For this review, take the finished solid that the model builds, in its own axes (mm). Round coordinates to 2 decimals unless told otherwise and drop trailing zeros. Write each loop counter-clockwise with the first axis right and the second up, starting at its lowest first coordinate (ties: lowest second). Pieces come first, ordered by that corner, then holes. Notation, with made-up numbers: M 11.25,60 L 56.25,60 A13 ccw 56.25,74 Z; hole C 84,32 d11. An arc over 180 degrees is marked long. Use one line per item in the form item = value. Start each with the question number.
Item 1: For line 1 (Y direction, x = -55, z = -0.85); line 2 (X direction, y = -1, z = -4.5); line 3 (Y direction, x = -48, z = -6.5), list the stretches that pass through material, from the lowest coordinate up. Write a range as [from, to].
Item 2: Add section C-C (z = -7.5). State the section outline as (x, y) points, and give its area (3 significant figures).
Item 3: Add section B-B (x = -19.5). State the section outline as (y, z) points, and give its area (3 significant figures).
Item 4: For P1, Ø5, axis at y = 2, z = -7.5, coming from the -X side; P2, Ø6, axis at x = -37.5, y = -3.5, coming from the +Z side; P3, Ø0.8, axis at x = 28.5, z = 0.5, coming from the -Y side, all flat-tipped, find the tip position at first contact; note any pin that passes through.
Item 5: Add section A-A (y = -1). State the section outline as (x, z) points.
Item 6: Add section D-D (y = 3.25). State the section outline as (x, z) points, and give its area (3 significant figures).
from build123d import *

# Parameters (mm, degrees)
F0_R     = 2.25
F0_W     = 15
F0_H     = 4.4
F1_DEPTH = 3
F2_DEPTH = 1.5
F4_DEPTH = 50


with BuildPart() as f1:
    # F0 (on Top) → F1 (new body)
    with BuildSketch(Plane.XY):
        with BuildLine():
            ThreePointArc((-50, 0), (-51.464466, 3.535534), (-55, 5))
            ThreePointArc((-55, 5), (-60, 0), (-55, -5))
            ThreePointArc((-55, -5), (-51.464466, -3.535534), (-50, 0))
        make_face()
        with Locations((-55, 0)):
            Circle(F0_R, mode=Mode.SUBTRACT)
        with BuildLine():
            ThreePointArc((55, -5), (50, 0), (55, 5))
            Line((55, 5), (-55, 5))
            ThreePointArc((-55, 5), (-51.464466, 3.535534), (-50, 0))
            ThreePointArc((-50, 0), (-51.464466, -3.535534), (-55, -5))
            Line((-55, -5), (55, -5))
        make_face()
        with Locations((-25, 0)):
            Rectangle(F0_W, F0_H, mode=Mode.SUBTRACT)
        with Locations((25, 0)):
            Rectangle(F0_W, F0_H, mode=Mode.SUBTRACT)
        with Locations((-25, 0)):
            Rectangle(F0_W, F0_H)
        with Locations((25, 0)):
            Rectangle(F0_W, F0_H)
        with BuildLine():
            ThreePointArc((55, -5), (58.535534, -3.535534), (60, 0))
            ThreePointArc((60, 0), (58.535534, 3.535534), (55, 5))
            ThreePointArc((55, 5), (50, 0), (55, -5))
        make_face()
        with Locations((55, 0)):
            Circle(F0_R, mode=Mode.SUBTRACT)
    extrude(amount=-F1_DEPTH)

    # F0 (on Top) → F2 (join)
    with BuildSketch(Plane.XY):
        with Locations((-25, 0)):
            Rectangle(F0_W, F0_H)
        with Locations((25, 0)):
            Rectangle(F0_W, F0_H)
    extrude(amount=F2_DEPTH)

    # F3 (on Right) → F4 (join, symmetric)
    with BuildSketch(Plane.YZ):
        Polygon((5, -3), (-5, -3), (-5, -13), align=None)
    extrude(amount=F4_DEPTH, both=True)


solid = f1.part
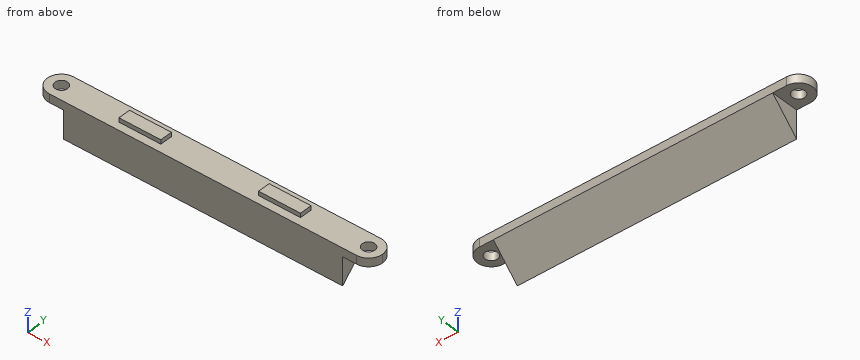
Calculated:
q1.line_1 = [-5, -2.25], [2.25, 5]
q1.line_2 = [-50, 50]
q1.line_3 = [-5, 1.5]
q2.outline = M -50,-5 L 50,-5 L 50,0.5 L -50,0.5 Z
q2.area = 550 mm^2
q3.outline = M -5,-13 L 5,-3 L 5,0 L 2.2,0 L 2.2,1.5 L -2.2,1.5 L -2.2,0 L -5,0 Z
q3.area = 86.6 mm^2
q4.P1 = -50
q4.P2 = 0
q4.P3 = -2.2
q5.outline = M -59.9,-3 L -57.02,-3 L -57.02,0 L -59.9,0 Z; M -52.98,-3 L -50,-3 L -50,-9 L 50,-9 L 50,-3 L 52.98,-3 L 52.98,0 L 32.5,0 L 32.5,1.5 L 17.5,1.5 L 17.5,0 L -17.5,0 L -17.5,1.5 L -32.5,1.5 L -32.5,0 L -52.98,0 Z; M 57.02,-3 L 59.9,-3 L 59.9,0 L 57.02,0 Z
q6.outline = M -58.8,-3 L -50,-3 L -50,-4.75 L 50,-4.75 L 50,-3 L 58.8,-3 L 58.8,0 L -58.8,0 Z
q6.area = 528 mm^2
